Design review of the part built by this model. Coordinates are the model's own, in mm. Give positions to 0.01 mm unless a question says otherwise; leave off trailing zeros. Loops run counter-clockwise (first coordinate to the right, second up) from the corner with the lowest first, then second, coordinate; pieces in that order, holes last. Notation, with made-up numbers: (22, 88) - (67, 88) arc R17 cw to (67, 112) - close; hole circle Ø7 at (76.25, 3). An arc over 180 degrees is marked (long way). Put each result on its own line as item: value. Start each with the question number.
```python
from build123d import *

# Parameters (mm, degrees)
F0_W     = 130
F0_H     = 130
F0_R     = 1.7
F1_DEPTH = 4
F2_R     = 5
F3_R     = 1
F4_SIZE  = 1.5


with BuildPart() as f1:
    # F0 (on Top) → F1 (new body)
    with BuildSketch(Plane.XY):
        Rectangle(F0_W, F0_H)
        with Locations((-49.5, -49.5)):
            Circle(F0_R, mode=Mode.SUBTRACT)
        with Locations((49.5, -49.5)):
            Circle(F0_R, mode=Mode.SUBTRACT)
        with Locations((-49.5, 49.5)):
            Circle(F0_R, mode=Mode.SUBTRACT)
        with Locations((49.5, 49.5)):
            Circle(F0_R, mode=Mode.SUBTRACT)
    extrude(amount=F1_DEPTH)

    # F2
    f2_edges = [f1.edges().sort_by_distance(p)[0] for p in [
        (65, 65, 2),
        (65, -65, 2),
        (-65, -65, 2),
        (-65, 65, 2),
    ]]
    fillet(f2_edges, radius=F2_R)

    # F3
    f3_edges = [f1.edges().sort_by_distance(p)[0] for p in [
        (65, 0, 4),
        (65, 0, 0),
    ]]
    fillet(f3_edges, radius=F3_R)

    # F4
    f4_edges = [f1.edges().sort_by_distance(p)[0] for p in [
        (-51.2, 49.5, 4),
        (47.8, 49.5, 4),
        (47.8, -49.5, 4),
        (-51.2, -49.5, 4),
    ]]
    chamfer(f4_edges, length=F4_SIZE)


solid = f1.part
```
Item 1: For L1, parallel to Y at x = 49.5, z = 1.85; L2, parallel to X at y = 58, z = 3.05; L3, parallel to Y at x = 0, z = 3.25, list the stretches that pass through material, from the lowest coordinate up. Write a range as from..to.
Item 2: Mouldability with a two-part tool opening along Y and no side actions: class faces 1 (the flat face through (-1, 1, 0)), 2 (the cylindrical face through (63, -64, 2)), 3 (the cylindrical face through (-50.85, -50.53, 1.23)) as pulls with the +Y half, pulls with the -Y half, needs draft (parallel to the pull), parting line crosses it, or undercut.
Item 3: Consider section A-A (x = 49.5). State the section outline as (y, z) points, plus the area to 3 significant figures.
Item 4: For P1, Ø1, axis at x = 35, y = -39.5, coming from the -Z side; P2, Ø4, axis at x = 49.5, y = -49.5, coming from the +Z side, all flat-tipped, find the tip position at first contact; note any pin that passes through.
Geometry says:
1. L1: y = -65..-51.2, -47.8..47.8, 51.2..65
1. L2: x = -65..65
1. L3: y = -64.97..64.97
2. face 1: needs draft
2. face 2: pulls with the -Y half
2. face 3: undercut
3. outline: (-65, 1) arc R1 ccw to (-64, 0) - (-51.2, 0) - (-51.2, 2.5) - (-52.7, 4) - (-64, 4) arc R1 ccw to (-65, 3) - close; (-47.8, 0) - (47.8, 0) - (47.8, 2.5) - (46.3, 4) - (-46.3, 4) - (-47.8, 2.5) - close; (51.2, 0) - (64, 0) arc R1 ccw to (65, 1) - (65, 3) arc R1 ccw to (64, 4) - (52.7, 4) - (51.2, 2.5) - close
3. area: 487 mm2
4. P1: stops at z = 0
4. P2: stops at z = 2.8
